Geometry: final body of the model. Coordinates: model frame, mm. Face numbers are marked on the shaded views. A direction names the side the tool comes from. Coordinates: 2 decimals unless noted, no trailing zeros. Loops run counter-clockwise (first coordinate to the right, second up) from the corner with the lowest first, then second, coordinate; pieces in that order, holes last. Notation, with made-up numbers: M 55,75 L 67,75 A17 ccw 67,103 Z; hole C 7.5,10 d8. An arc over 180 degrees is marked long. Write item = value, one per line. Start each with the question number.
```python
from build123d import *

# Parameters (mm, degrees)
SKETCH1_W                     = 7.5
SKETCH1_H                     = 7.5
BOSS_EXTRUDE1_DEPTH           = 7
SKETCH2_W                     = 13
SKETCH2_H                     = 13
BOSS_EXTRUDE2_DEPTH           = 3.8
SKETCH3_W                     = 6
SKETCH3_H                     = 6
CUT_EXTRUDE1_DEPTH            = 11.8
SKETCH6_W                     = 12
SKETCH6_H                     = 12
CUT_EXTRUDE3_DEPTH            = 2.8
FILLET1_R                     = 0.5
BOSS_EXTRUDE3_REACH           = 12.8
FILLET4_R                     = 1.5
FILLET2_R                     = 1
TAP_DRILL_FOR_0_80_TAP1_D     = 1.19126
TAP_DRILL_FOR_0_80_TAP1_DEPTH = 7.11
TAP_DRILL_FOR_0_80_TAP1_TIP   = 0.357890611
FILLET5_R                     = 2.25
SKETCH16_W                    = 2.5
SKETCH16_H                    = 2
CUT_EXTRUDE4_DEPTH            = 0.835786
FILLET6_R                     = 1


with BuildPart() as part:
    # Sketch1 → Boss-Extrude1 (new body)
    with BuildSketch(Plane(origin=(0, 0, 0), x_dir=(1, 0, 0), z_dir=(0, 1, 0))):
        Rectangle(SKETCH1_W, SKETCH1_H)
    extrude(amount=BOSS_EXTRUDE1_DEPTH)

    # Sketch2 → Boss-Extrude2 (add)
    with BuildSketch(Plane(origin=(0, 7, 0), x_dir=(1, 0, 0), z_dir=(0, 1, 0))):
        Rectangle(SKETCH2_W, SKETCH2_H)
    extrude(amount=BOSS_EXTRUDE2_DEPTH)

    # Sketch3 → Cut-Extrude1 (cut, through all)
    with BuildSketch(Plane.XZ):
        Rectangle(SKETCH3_W, SKETCH3_H)
    extrude(amount=-CUT_EXTRUDE1_DEPTH, mode=Mode.SUBTRACT)

    # Sketch6 → Cut-Extrude3 (cut)
    with BuildSketch(Plane(origin=(0, 10.8, 0), x_dir=(1, 0, 0), z_dir=(0, 1, 0))):
        Rectangle(SKETCH6_W, SKETCH6_H)
    extrude(amount=-CUT_EXTRUDE3_DEPTH, mode=Mode.SUBTRACT)

    # Fillet1
    fillet1_edges = [part.edges().sort_by_distance(p)[0] for p in [
        (6, 9.4, 6),
        (6, 9.4, -6),
        (-6, 9.4, -6),
        (-6, 9.4, 6),
    ]]
    fillet(fillet1_edges, radius=FILLET1_R)

    # Sketch12 → Boss-Extrude3 (add, up to next)
    with BuildSketch(Plane.XZ, mode=Mode.PRIVATE) as boss_extrude3_sk1:
        Polygon((3.75, -3.75), (4.633883476, -2.866116524), (3.75, -1.982233047), align=None)
    boss_extrude3_tool1 = extrude(boss_extrude3_sk1.sketch, amount=-BOSS_EXTRUDE3_REACH, mode=Mode.PRIVATE) - part.part
    add(boss_extrude3_tool1.solids().sort_by_distance((4.044628, 0, -2.866117))[0])
    # Sketch12 → Boss-Extrude3 (add, up to next)
    with BuildSketch(Plane.XZ, mode=Mode.PRIVATE) as boss_extrude3_sk2:
        Polygon((2.866116524, -4.633883476), (3.75, -3.75), (1.982233047, -3.75), align=None)
    boss_extrude3_tool2 = extrude(boss_extrude3_sk2.sketch, amount=-BOSS_EXTRUDE3_REACH, mode=Mode.PRIVATE) - part.part
    add(boss_extrude3_tool2.solids().sort_by_distance((2.866117, 0, -4.044628))[0])

    # Fillet4
    fillet4_edges = [part.edges().sort_by_distance(p)[0] for p in [
        (-3, 4, 3),
        (3, 4, 3),
        (-3, 4, -3),
        (3, 4, -3),
    ]]
    fillet(fillet4_edges, radius=FILLET4_R)

    # Fillet2
    fillet2_edges = [part.edges().sort_by_distance(p)[0] for p in [
        (3.75, 3.5, -1.982233047),
        (1.982233047, 3.5, -3.75),
    ]]
    fillet(fillet2_edges, radius=FILLET2_R)

    # Tap Drill for #0-80 Tap1
    with Locations(Plane(origin=(3.75, 0, -3.75), x_dir=(-0.707106781, 0, -0.707106781), z_dir=(0.707106781, 0, -0.707106781))):
        with Locations((0, 1.25), (0, 3.75)):
            Hole(TAP_DRILL_FOR_0_80_TAP1_D / 2, depth=TAP_DRILL_FOR_0_80_TAP1_DEPTH)
            with Locations((0, 0, -(TAP_DRILL_FOR_0_80_TAP1_DEPTH + TAP_DRILL_FOR_0_80_TAP1_TIP / 2))):  # 118° drill point
                Cone(0, TAP_DRILL_FOR_0_80_TAP1_D / 2, TAP_DRILL_FOR_0_80_TAP1_TIP, mode=Mode.SUBTRACT)

    # Fillet5
    fillet5_edges = [part.edges().sort_by_distance(p)[0] for p in [
        (3.75, 3.5, 3.75),
        (-3.75, 3.5, 3.75),
        (-3.75, 3.5, -3.75),
    ]]
    fillet(fillet5_edges, radius=FILLET5_R)

    # Sketch16 → Cut-Extrude4 (cut)
    with BuildSketch(Plane(origin=(3.75, 0, -3.75), x_dir=(-0.707106781, 0, -0.707106781), z_dir=(0.707106781, 0, -0.707106781))):
        with Locations((0, 6)):
            Rectangle(SKETCH16_W, SKETCH16_H)
    extrude(amount=-CUT_EXTRUDE4_DEPTH, mode=Mode.SUBTRACT)

    # Fillet6
    fillet6_edges = [part.edges().sort_by_distance(p)[0] for p in [
        (-6.5, 8.9, -6.5),
        (-6.5, 8.9, 6.5),
        (6.5, 8.9, 6.5),
        (6.5, 8.9, -6.5),
    ]]
    fillet(fillet6_edges, radius=FILLET6_R)


solid = part.part
```
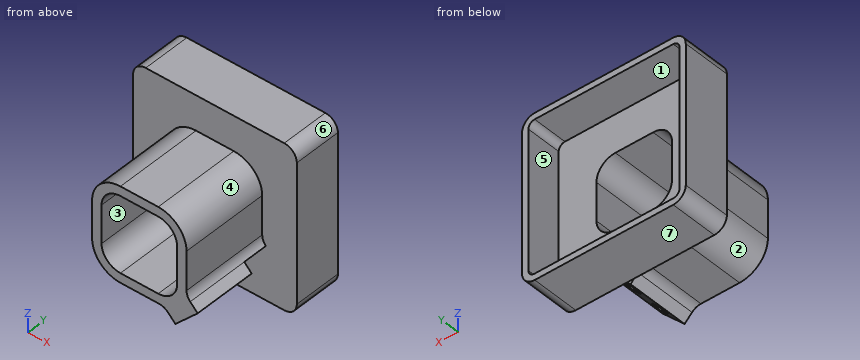
Item 1: Section query D-D (y = 9.75). Return the cut outline in (x, z), plus the area to 3 significant figures.
Item 2: Section query C-C (z = -1). Return the cut outline in (x, y).
Item 3: First-contact query: pin 1 (1.9 mm diameter, centred on x = 3.5, z = -4, fed in from +Y); pin 2 (1 mm diameter, centred on y = 2.5, z = -1.5, fed in from +X); pin 3 (1.5 mm diameter, centred on x = 0.5, y = 5.5, fed in from -Z). Flat tips, straight axial feed; report the tip coordinate or a pass-through.
Item 4: Reachability of the marked faces 1, 2, 3 and 4 from +Z, -Z, +X, -X, +Y, -Y: full face, straight path, thin tool, end or side. Return the list, or none.
Item 5: Line query: line 1 (Z direction, x = 0.25, y = 1); line 2 (X direction, y = 9, z = 4.75); line 3 (X direction, y = 7.5, z = 0). Output: solid intervals per line, ascending. Write a range as from..to.
Item 6: Pull-direction query (X, two-part tool) for the marked faces 5, 6 and 7; classes: released by +X, released by -X, zero draft, split by the parting line, or undercut.
Item 7: Section query A-A (y = 6). Return the cut outline in (x, z), plus the area to 3 significant figures.
Item 8: Section query B-B (x = 1). Return the cut outline in (y, z).
Verdict:
q1.outline = M -6.5,-5.5 A1 ccw -5.5,-6.5 L 5.5,-6.5 A1 ccw 6.5,-5.5 L 6.5,5.5 A1 ccw 5.5,6.5 L -5.5,6.5 A1 ccw -6.5,5.5 Z; hole M -6,-5.5 A0.5 ccw -5.5,-6 L 5.5,-6 A0.5 ccw 6,-5.5 L 6,5.5 A0.5 ccw 5.5,6 L -5.5,6 A0.5 ccw -6,5.5 Z
q1.area = 24.4 mm2
q2.outline = M -6.5,7 L -3.75,7 L -3.75,0 L -3,0 L -3,8 L -6,8 L -6,10.8 L -6.5,10.8 Z; M 3,0 L 3.75,0 L 3.75,7 L 6.5,7 L 6.5,10.8 L 6,10.8 L 6,8 L 3,8 Z
q3.pin_1 = 8
q3.pin_2 = 3.85
q3.pin_3 = -3.75
q4.face_1 = +Y
q4.face_2 = -Z, -X, -Y
q4.face_3 = +Y, -Y
q4.face_4 = +Z, +X, -Y
q5.line_1 = -3.75..-3, 3..3.75
q5.line_2 = -6.5..-6, 6..6.5
q5.line_3 = -6.5..-3, 3..6.5
q6.face_5 = undercut
q6.face_6 = released by +X
q6.face_7 = zero draft
q7.outline = M -3.75,-1.5 A2.25 ccw -1.5,-3.75 L 1.57,-3.75 A1 cw 2.28,-4.04 L 4.04,-2.28 A1 cw 3.75,-1.57 L 3.75,1.5 A2.25 ccw 1.5,3.75 L -1.5,3.75 A2.25 ccw -3.75,1.5 Z; hole M -3,-1.5 A1.5 ccw -1.5,-3 L 1.5,-3 A1.5 ccw 3,-1.5 L 3,1.5 A1.5 ccw 1.5,3 L -1.5,3 A1.5 ccw -3,1.5 Z
q7.area = 18.4 mm2
q8.outline = M 0,-3.75 L 7,-3.75 L 7,-6.5 L 10.8,-6.5 L 10.8,-6 L 8,-6 L 8,-3 L 0,-3 Z; M 0,3 L 8,3 L 8,6 L 10.8,6 L 10.8,6.5 L 7,6.5 L 7,3.75 L 0,3.75 Z
